Geometry: final body of the model. Coordinates: model frame, mm. Give positions to 0.01 mm unless a question says otherwise; leave off trailing zeros. Loops run counter-clockwise (first coordinate to the right, second up) from the corner with the lowest first, then second, coordinate; pieces in that order, holes last.
Autodesk Inventor part; units mm, degrees
ref_plane "YZ Plane" through (0, 0, 0) normal (1, 0, 0) x (0, 1, 0)
ref_plane "XZ Plane" through (0, 0, 0) normal (0, 1, 0) x (-1, 0, 0)
ref_plane "XY Plane" through (0, 0, 0) normal (0, 0, 1) x (1, 0, 0)
sketch "Sketch1" plane through (0, 0, 0) normal (0, 1, 0) x (-1, 0, 0)
  line L0 (53.5, 75) -> (-53.5, 75)
  line L1 (-53.5, 75) -> (-53.5, -75)
  line L2 (-53.5, -75) -> (53.5, -75)
  line L3 (53.5, -75) -> (53.5, 75)
  line L4 (74.9, 0) -> (-74.9, 0)
  line L5 (0, -105) -> (0, 105)
  point P0 (0, 0)
  point P1 (0, 75)
  point P2 (53.5, 0)
  dimension "d0" = 150
  dimension "d1" = 107
extrude "Extrusion1" add sketch "Sketch1" along normal blind 3.175
sketch "Sketch2" plane through (0, 3.175, 0) normal (0, 1, 0) x (1, 0, 0)
  line L0 (-53.5, -75) -> (53.5, -75)
  line L1 (-53.5, 75) -> (-53.5, -75)
  line L2 (53.5, 75) -> (-53.5, 75)
  line L3 (0, 105) -> (0, -105)
  line L4 (-20.25, -70) -> (20.25, -70) construction
  line L5 (20.25, -70) -> (20.25, 70) construction
  line L6 (20.25, 70) -> (-20.25, 70) construction
  line L7 (-20.25, 70) -> (-20.25, -70) construction
  line L8 (-6, -6) -> (6, -6) construction
  line L9 (6, -6) -> (6, 6) construction
  line L10 (6, 6) -> (-6, 6) construction
  line L11 (-6, 6) -> (-6, -6) construction
  line L12 (-43.5, -65) -> (43.5, -65) construction
  line L13 (43.5, -65) -> (43.5, 65) construction
  line L14 (43.5, 65) -> (-43.5, 65) construction
  line L15 (-43.5, 65) -> (-43.5, -65) construction
  line L16 (-17.5, -10.5) -> (17.5, -10.5) construction
  line L17 (-74.9, 0) -> (74.9, 0)
  point P0 (0, -10.5)
  point P1 (0, -6)
  point P2 (-6, 0)
  point P3 (0, -65)
  point P4 (-43.5, 0)
  point P5 (-20.25, 0)
  point P6 (0, -70)
  dimension "d31" = 64.5
  dimension "d32" = 12
  dimension "d33" = 12
  dimension "d34" = 35
  dimension "d35" = 10
  dimension "d36" = 10
  dimension "d37" = 5
  dimension "d38" = 40.5
hole "Hole3" at (-43.5, 3.175, 65) at (-20.25, 3.175, 70) at (20.25, 3.175, 70) at (43.5, 3.175, 65) at (43.5, 3.175, -65) at (20.25, 3.175, -70) at (-20.25, 3.175, -70) at (-43.5, 3.175, -65) at (-17.5, 3.175, 10.5) at (17.5, 3.175, 10.5) direction (0, -1, 0) diameter 4 end through all
hole "Hole4" at (-6, 3.175, 6) at (-6, 3.175, -6) at (6, 3.175, 6) at (6, 3.175, -6) direction (0, -1, 0) diameter 3 end through all
equation "\"d36\" = d35"
properties part number "base superior"
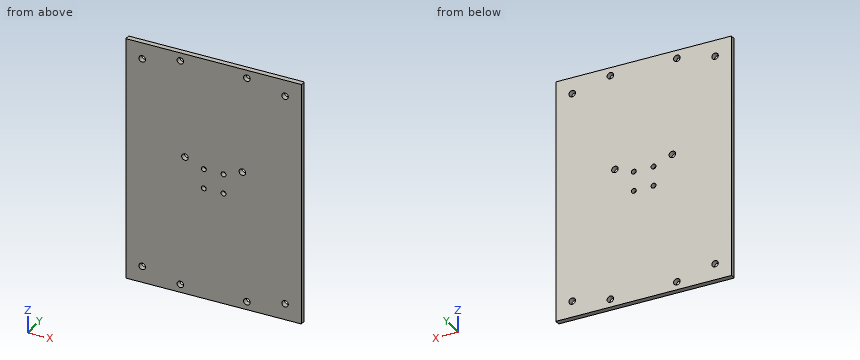
Q1. Pin query (flat end, axial travel): pin 1 Ø5 at (x, z) = (43.5, 65) entering from -Y; pin 2 Ø2.5 at (x, z) = (6, -6) entering from +Y. Return the tip coordinate at first contact, or that it passes through.
Q2. Material intervals for probe 1 along Z at (x, y) = (-6, 1.4); probe 2 along X at (y, z) = (2.45, -70); probe 3 along Z at (x, y) = (-20.25, 2.45), sorted ascending.
Q3. Section query A-A, the plane x = 43.5. Return loops of the section in (y, z) (3 decimals).
Q4. Section query B-B, the plane z = -6. Return loops of the section in (x, y) (3 decimals), and give its area (3 significant figures).
Resolved:
1. pin 1: stops at y = 0
1. pin 2: passes through
2. probe 1: z = -75 to -7.5, -4.5 to 4.5, 7.5 to 75
2. probe 2: x = -53.5 to -22.25, -18.25 to 18.25, 22.25 to 53.5
2. probe 3: z = -75 to -72, -68 to 68, 72 to 75
3. outline: (0, -75) - (3.175, -75) - (3.175, -67) - (0, -67) - close; (0, -63) - (3.175, -63) - (3.175, 63) - (0, 63) - close; (0, 67) - (3.175, 67) - (3.175, 75) - (0, 75) - close
4. outline: (-53.5, 0) - (-7.5, 0) - (-7.5, 3.175) - (-53.5, 3.175) - close; (-4.5, 0) - (4.5, 0) - (4.5, 3.175) - (-4.5, 3.175) - close; (7.5, 0) - (53.5, 0) - (53.5, 3.175) - (7.5, 3.175) - close
4. area: 321 mm2
